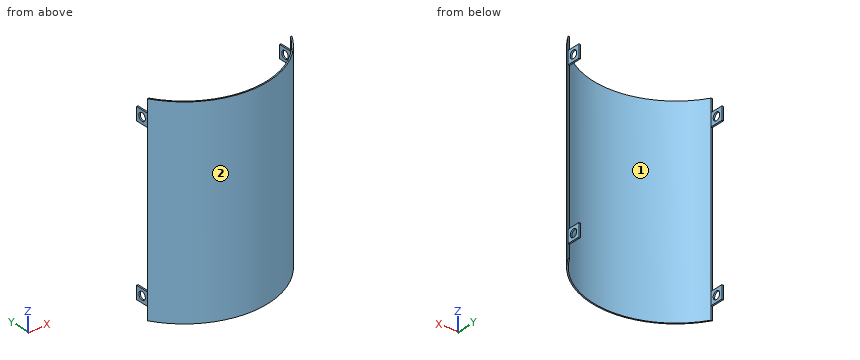
Autodesk Inventor part; units mm, degrees
ref_plane "YZ Plane" through (0, 0, 0) normal (1, 0, 0) x (0, 1, 0)
ref_plane "XZ Plane" through (0, 0, 0) normal (0, 1, 0) x (-1, 0, 0)
ref_plane "XY Plane" through (0, 0, 0) normal (0, 0, 1) x (1, 0, 0)
sketch "Szkic1" plane through (0, 0, 0) normal (0, 0, 1) x (1, 0, 0)
  circle A0 centre (0, 0) radius 32.5
  circle A1 centre (0, 0) radius 32
  dimension "d0" = 65
  dimension "d1" = 64
extrude "Wyciągnięcie proste1" add sketch "Szkic1" along normal blind 77
sketch "Szkic2" plane through (0, 0, 77) normal (0, 0, 1) x (1, 0, 0)
  line L0 (0, 0) -> (-28, 0)
  line L1 (-28, 0) -> (-28, 15.4919)
  circle A0 centre (0, 0) radius 32
  line L2 (-28, 0) -> (-28, -16.5)
  circle A1 centre (0, 0) radius 32.5
  line L3 (-28, -16.5) -> (28, -16.5)
  line L4 (52.8927, -0.6882) -> (26.703, 44.9724)
  line L5 (26.703, 44.9724) -> (-31.7097, 42.3671)
  line L6 (-31.7097, 42.3671) -> (-48.5067, -13.9887)
  line L7 (-48.5067, -13.9887) -> (-28, -16.5)
  line L8 (28, -16.5) -> (52.8927, -0.6882)
  dimension "d4" = 28
extrude "Wyciągnięcie proste2" cut sketch "Szkic2" against normal blind 77 contours L2 A0 L1 | L1 A0 L3 L2 | A0 L2 A1 L3 | A0 L3 L2 | L7 L6 L5 L4 L8 A1
sketch "Szkic3" plane through (-27.4181, -16.5, 77) normal (0, 1, 0) x (1, 0, 0)
  line L0 (-0.5819, 0) -> (55.4181, 0)
  line L1 (-0.5819, 0) -> (-0.5819, 5)
  line L2 (-0.5819, 0) -> (-0.5819, 77)
  line L3 (-0.5819, 5) -> (0, 5)
  line L4 (0, 77) -> (0, 0)
  line L5 (0, 5) -> (0, 10)
  line L6 (0, 10) -> (-0.5819, 10)
  line L7 (-0.5819, 10) -> (-0.5819, 5)
  line L8 (-0.5819, 77) -> (55.4181, 77)
  line L9 (-0.5819, 77) -> (-0.5819, 72)
  line L10 (-0.5819, 72) -> (0, 72)
  line L11 (0, 72) -> (0, 67)
  line L12 (0, 67) -> (-0.5819, 67)
  line L13 (-0.5819, 67) -> (-0.5819, 72)
  line L14 (55.4181, 77) -> (55.4181, 72)
  line L15 (55.4181, 77) -> (55.4181, 0)
  line L16 (55.4181, 72) -> (54.8361, 72)
  line L17 (54.8361, 0) -> (54.8361, 77)
  line L18 (54.8361, 72) -> (54.8361, 67)
  line L19 (54.8361, 67) -> (55.4181, 67)
  line L20 (55.4181, 67) -> (55.4181, 72)
  line L21 (55.4181, 0) -> (55.4181, 5)
  line L22 (55.4181, 5) -> (54.8361, 5)
  line L23 (54.8361, 5) -> (54.8361, 10)
  line L24 (54.8361, 10) -> (55.4181, 10)
  line L25 (55.4181, 10) -> (55.4181, 5)
  point P0 (27.4181, 77)
  dimension "d7" = 5
  dimension "d8" = 5
  dimension "d9" = 5
  dimension "d10" = 5
  dimension "d11" = 5
  dimension "d12" = 5
  dimension "d13" = 5
  dimension "d14" = 5
extrude "Wyciągnięcie proste3" add sketch "Szkic3" along normal blind 5 contours L2 L6 L4 L3 | L17 L24 L15 L22 | L2 L10 L4 L12 | L17 L16 L15 L19
sketch "Szkic4" plane through (28, -16.5, 67) normal (1, 0, 0) x (0, 0, -1)
  line L0 (57, 0) -> (57, 5)
  line L1 (62, 0) -> (62, 5)
  line L2 (57, 0) -> (62, 5)
  line L3 (62, 5) -> (57, 5)
  line L4 (62, 5) -> (57, 5)
  line L5 (57, 5) -> (62, 0)
  line L6 (0, 0) -> (-5, 0)
  line L7 (-5, 5) -> (0, 5)
  line L8 (-5, 0) -> (0, 5)
  line L9 (0, 5) -> (-5, 5)
  line L10 (-5, 5) -> (0, 0)
  circle A0 centre (-2.5, 2.5) radius 1.5
  circle A1 centre (59.5, 2.5) radius 1.5
  point P0 (67, 16.5)
  dimension "d17" = 3
  dimension "d18" = 3
extrude "Wyciągnięcie proste4" cut sketch "Szkic4" against normal up to surface (56 mm away) contours A1 L5 L2 | L2 L5 A1 | A1 L2 L5 | L2 A1 L5 | A0 L8 L10 | L10 L8 A0 | A0 L10 L8 | L10 A0 L8
properties part number "Obudowa, większa"
The listing builds one solid part. Answer for the finished solid, in the listing's coordinates (mm). Face numbers are marked on the shaded views. Give positions to 0.01 mm unless a question says otherwise; leave off trailing zeros. Loops run counter-clockwise (first coordinate to the right, second up) from the corner with the lowest first, then second, coordinate; pieces in that order, holes last.
Item 1: A cutting plane is placed at A-A (y = -22). Give the vertices of the cut face in (x, z), then the cut area to 3 significant figures.
Derived:
outline: (-23.92, 0) - (-23.24, 0) - (-23.24, 77) - (-23.92, 77) - close; (23.24, 0) - (23.92, 0) - (23.92, 77) - (23.24, 77) - close
area: 105 mm2
Item 2: A cutting plane is placed at D-D (y = -17.5). Give the vertices of the cut face in (x, z), then the cut area to 3 significant figures.
Derived:
outline: (-27.39, 0) - (-26.79, 0) - (-26.79, 77) - (-27.39, 77) - close; (26.79, 0) - (27.39, 0) - (27.39, 77) - (26.79, 77) - close
area: 91.7 mm2
Item 3: Each of these flat-tipped pins is pushed along its axis until it touches: pin 1 Ø8 at (x, z) = (-4, 29) entering from +Y; pin 2 Ø6 at (y, z) = (-27, 11) entering from +X; pin 3 Ø1.5 at (y, z) = (-24, 11) entering from +X. Where does it stop, or does it pass through?
Derived:
pin 1: stops at y = -30.98
pin 2: stops at x = 21.91
pin 3: stops at x = 22.71
Item 4: A cutting plane is placed at B-B (z = 69.5). Give the number of separate pieces and of enclosed holes in the cut face, then the cut area to 3 significant figures.
Derived:
separate pieces: 3
enclosed holes: 0
area: 35.7 mm2
Item 5: Determine the mould class of the marked faces 1 and 2 for opening direction X: +X half, -X half, draft (parallel to the pull), parting line (faces both ways), or undercut.
Derived:
face 1: undercut
face 2: parting line
Item 6: Find the intervals of material crossed by line 1 along Z through (x, y) = (27.65, -14); line 2 along X through (y, z) = (-28, 66.5); line 3 along X through (y, z) = (-17.75, 14), in increasing order.
Derived:
line 1: z = 5 to 6, 9 to 10, 67 to 68, 71 to 72
line 2: x = -16.5 to -15.49, 15.49 to 16.5
line 3: x = -27.22 to -26.63, 26.63 to 27.22
